```python
from build123d import *

# Parameters (mm, degrees)
EXTRUDE_1_DEPTH          = 1
EXTRUDE_2_DEPTH          = 1
SKETCH_5_W               = 95.882599
SKETCH_5_H               = 27.8428
EXTRUDE_3_DEPTH          = 2
CUT_EXTRUDE_1_DEPTH      = 100.923442209
CUT_EXTRUDE_1_DEPTH_BACK = 100.923442209
SKETCH_6_R               = 5
CUT_EXTRUDE_2_DEPTH      = 100.923442209
CUT_EXTRUDE_2_DEPTH_BACK = 100.923442209
SKETCH_7_R               = 1.35
SKETCH_8_W               = 95.882599
SKETCH_8_H               = 20
EXTRUDE_4_DEPTH          = 2
EXTRUDE_5_DEPTH          = 1
SKETCH_10_W              = 40
SKETCH_10_H              = 120
EXTRUDE_6_DEPTH          = 2
EXTRUDE_START            = -3
EXTRUDE_7_DEPTH          = 3
SKETCH_12_W              = 5
SKETCH_12_H              = 123
EXTRUDE_8_DEPTH          = 1
EXTRUDE_9_OUTLINE_W      = 95.901549254
EXTRUDE_9_OUTLINE_H      = 3
EXTRUDE_9_OUTLINE_W_2    = 95.885
EXTRUDE_9_OUTLINE_H_2    = 2
EXTRUDE_9_DEPTH          = 2
EXTRUDE_START_2          = -1
EXTRUDE_9_2_OUTLINE_W    = 95.885
EXTRUDE_9_2_OUTLINE_H    = 2
EXTRUDE_9_2_DEPTH        = 1
CUT_EXTRUDE_3_DEPTH      = 177.247383378
CUT_EXTRUDE_3_DEPTH_BACK = 177.247383378
SKETCH_16_R              = 1.35
SKETCH_17_W              = 30
SKETCH_17_H              = 70
EXTRUDE_10_DEPTH         = 2
EXTRUDE_11_DEPTH         = 3


# Read off the part's stored shape, not the designer's step: 凸台-拉伸9
with BuildPart() as part:
    # 草图3 → 凸台-拉伸1 (new body)
    with BuildSketch(Plane(origin=(0, 0, 0), x_dir=(1, 0, 0), z_dir=(0, 1, 0))):
        with BuildLine():
            Line((41.882488294, 21.631498957), (31.610829647, 15.243028334))
            ThreePointArc((31.610829647, 15.243028334), (31.350600602, 14.569512784), (31.613242469, 13.896934459))
            Line((31.613242469, 13.896934459), (40.546880152, 8.234769731))
            ThreePointArc((40.546880152, 8.234769731), (44.573930655, 7.017936995), (48.601204689, 8.234029718))
            Line((48.601204689, 8.234029718), (57.364385058, 13.822144736))
            ThreePointArc((57.364385058, 13.822144736), (57.798599734, 14.63340346), (57.366705056, 15.44589967))
            Line((57.366705056, 15.44589967), (47.51874726, 21.632437259))
            ThreePointArc((47.51874726, 21.632437259), (44.700511427, 22.270800367), (41.882488294, 21.631498957))
        make_face()
    extrude(amount=EXTRUDE_1_DEPTH)

    # 草图4 → 凸台-拉伸2 (add)
    with BuildSketch(Plane.XZ):
        with BuildLine():
            Line((49.96883361, -25.998027869), (60.064619869, -19.655803167))
            ThreePointArc((60.064619869, -19.655803167), (62.798594558, -14.643390815), (60.079038247, -9.623140954))
            Line((60.079038247, -9.623140954), (51.324268762, -4.040389399))
            ThreePointArc((51.324268762, -4.040389399), (44.577632655, -2.01793734), (37.829997654, -4.03705422))
            Line((37.829997654, -4.03705422), (28.614522584, -9.877848279))
            ThreePointArc((28.614522584, -9.877848279), (26.350608769, -14.582124379), (28.631489707, -19.27819737))
            Line((28.631489707, -19.27819737), (39.443234024, -26.002574933))
            ThreePointArc((39.443234024, -26.002574933), (44.706582673, -27.270799381), (49.96883361, -25.998027869))
        make_face()
    extrude(amount=EXTRUDE_2_DEPTH)

    # 草图5 → 凸台-拉伸3 (add)
    with BuildSketch(Plane.XZ.offset(1)):
        with Locations((47.9412995, -13.9214)):
            Rectangle(SKETCH_5_W, SKETCH_5_H)
    extrude(amount=EXTRUDE_3_DEPTH)

    # 草图6 → 切除-拉伸1 (cut, two sides: drawn at the far end of the back side and taken through both)
    with BuildSketch(Plane.XZ.offset(3).offset(-CUT_EXTRUDE_1_DEPTH_BACK)):
        with Locations(Location((16.25, -19.8, 0), (0, 0, 270))):
            Circle(SKETCH_6_R)
    extrude(amount=CUT_EXTRUDE_1_DEPTH + CUT_EXTRUDE_1_DEPTH_BACK, mode=Mode.SUBTRACT)

    # 草图7 → 切除-拉伸2 (cut, two sides: drawn at the far end of the back side and taken through both)
    with BuildSketch(Plane(origin=(0, 1, 0), x_dir=(1, 0, 0), z_dir=(0, 1, 0)).offset(-CUT_EXTRUDE_2_DEPTH_BACK)):
        with Locations(Location((37.074600168, 14.583340303, 0), (0, 0, 270))):
            Circle(SKETCH_7_R)
        with Locations(Location((52.074600168, 14.619575942, 0), (0, 0, 270))):
            Circle(SKETCH_7_R)
    extrude(amount=CUT_EXTRUDE_2_DEPTH + CUT_EXTRUDE_2_DEPTH_BACK, mode=Mode.SUBTRACT)

    # 草图8 → 凸台-拉伸4 (add)
    with BuildSketch(Plane(origin=(0, -1, 0), x_dir=(1, 0, 0), z_dir=(0, 1, 0))):
        with Locations((47.9412995, -10)):
            Rectangle(SKETCH_8_W, SKETCH_8_H)
    extrude(amount=-EXTRUDE_4_DEPTH)

    # 草图9 → 凸台-拉伸5 (add)
    with BuildSketch(Plane(origin=(0, -1, 0), x_dir=(1, 0, 0), z_dir=(0, 1, 0))):
        Polygon((0, 0), (0, 4), (95.882599, 4), (95.882599, 0), (95.898271126, -2), (-0.002401, -2), align=None)
    extrude(amount=EXTRUDE_5_DEPTH)

    # 草图10 → 凸台-拉伸6 (add)
    with BuildSketch(Plane(origin=(0, -1, 0), x_dir=(1, 0, 0), z_dir=(0, 1, 0))):
        with Locations((75.882599, 87.8428)):
            Rectangle(SKETCH_10_W, SKETCH_10_H)
    extrude(amount=-EXTRUDE_6_DEPTH)

    # 草图11 → 凸台-拉伸7 (add)
    with BuildSketch(Plane.XZ.offset(3).offset(EXTRUDE_START)):
        Polygon((-0.002401, -27.8428), (-0.002401, -30.8428), (55.882599, -30.8428), (55.882599, -27.8428), (55.882599, -24.8428), (0, -24.8428), align=None)
    extrude(amount=EXTRUDE_7_DEPTH)

    # 草图12 → 凸台-拉伸8 (add)
    with BuildSketch(Plane(origin=(0, -1, 0), x_dir=(1, 0, 0), z_dir=(0, 1, 0))):
        with Locations((58.382599, 86.3428)):
            Rectangle(SKETCH_12_W, SKETCH_12_H)
    extrude(amount=EXTRUDE_8_DEPTH)

    # 凸台-拉伸9 outline → 凸台-拉伸9 (add)
    with BuildSketch(Plane(origin=(0, 0, 0), x_dir=(1, 0, 0), z_dir=(0, 1, 0))):
        with Locations((47.948373627, -2.4702)):
            Rectangle(EXTRUDE_9_OUTLINE_W, EXTRUDE_9_OUTLINE_H)
        with Locations((47.940099, 29.8428)):
            Rectangle(EXTRUDE_9_OUTLINE_W_2, EXTRUDE_9_OUTLINE_H_2)
    extrude(amount=EXTRUDE_9_DEPTH)

    # Extrude 9 2 outline → Extrude 9 2 (add)
    with BuildSketch(Plane(origin=(0, 0, 0), x_dir=(1, 0, 0), z_dir=(0, 1, 0)).offset(EXTRUDE_START_2)):
        with Locations((47.940099, 29.8428)):
            Rectangle(EXTRUDE_9_2_OUTLINE_W, EXTRUDE_9_2_OUTLINE_H)
    extrude(amount=EXTRUDE_9_2_DEPTH)

    # 草图16 → 切除-拉伸3 (cut, two sides: drawn at the far end of the back side and taken through both)
    with BuildSketch(Plane(origin=(0, -1, 0), x_dir=(1, 0, 0), z_dir=(0, 1, 0)).offset(-CUT_EXTRUDE_3_DEPTH_BACK)):
        with Locations(Location((19.997599, -10, 0), (0, 0, 270))):
            Circle(SKETCH_16_R)
        with Locations(Location((26.997599, -10, 0), (0, 0, 270))):
            Circle(SKETCH_16_R)
    extrude(amount=CUT_EXTRUDE_3_DEPTH + CUT_EXTRUDE_3_DEPTH_BACK, mode=Mode.SUBTRACT)

    # 草图17 → 凸台-拉伸10 (add)
    with BuildSketch(Plane(origin=(0, -1, 0), x_dir=(1, 0, 0), z_dir=(0, 1, 0))):
        with Locations((110.882599, 112.8428)):
            Rectangle(SKETCH_17_W, SKETCH_17_H)
    extrude(amount=-EXTRUDE_10_DEPTH)

    # 草图18 → 凸台-拉伸11 (add)
    with BuildSketch(Plane(origin=(0, -1, 0), x_dir=(1, 0, 0), z_dir=(0, 1, 0))):
        Polygon((95.882599, 30.8428), (95.882599, 77.8428), (125.882599, 77.8428), (125.882599, 80.8428), (92.882599, 80.8428), (92.882599, 31.8428), (60.882599, 31.8428), (60.882599, 144.8428), (125.882599, 144.8428), (125.882599, 147.8428), (55.882599, 147.8428), (55.882599, 30.8428), (60.882599, 30.8428), align=None)
    extrude(amount=EXTRUDE_11_DEPTH)


solid = part.part
```
Check sheet for the modelled part. Datum: model origin and axes. Units: mm. A direction names the side the tool comes from. Give positions to 0.01 mm unless a question says otherwise; leave off trailing zeros. Loops run counter-clockwise (first coordinate to the right, second up) from the corner with the lowest first, then second, coordinate; pieces in that order, holes last. Notation, with made-up numbers: (-6, -28.5) - (28, -28.5) arc R16 cw to (28, -5.5) - close; hole circle Ø9 at (3.25, 49). An arc over 180 degrees is marked (long way). One line per question, with ' | ' between items. Start each with the question number.
1. Gauge pin test, flat ends, axial feed: pin 1 Ø6 at (x, z) = (16.25, -19.8) entering from +Y; pin 2 Ø2.5 at (x, y) = (37.5, -1) entering from -Z; pin 3 Ø20 at (x, z) = (83.5, -18.5) entering from +Y; pin 4 Ø1.5 at (y, z) = (-1.5, -87) entering from -X. Record the tip position at first contact, or that the pin passes through.
2. Draft check along Z on faces 1 (the flat face through (52.92, 0.49, -10.99)), 2 (the flat face through (91, -1, -147.843)), 3 (the flat face through (76, -3, -65)). Enter one of: released by +Z, released by -Z, zero draft, split by the parting line, or undercut.
3. Cross-section at C-C, the plane x = 108.5. Enter the section's corners in (y, z).
4. Cross-section at A-A, the plane x = 16.25. Enter the section's corners in (y, z).
5. Cross-section at B-B, the plane z = -72. Enter the section's corners in (x, y).
6. Set-up check for faces 4 (the flat face through (52.512, 0.493, -18.496)), 5 (the flat face through (111, -1, -77.843)), 6 (the flat face through (44, 1, -15)), 7 (the flat face through (36.819, 0.493, -18.482)), 8 (the flat face through (55.883, -1, -90)): record each of +Z, -Z, +X, -X, +Y, -Y from which the full face is reachable in a straight line by a thin tool's end or side.
7. Material ranges on line 1 along Z through (x, y) = (56.5, 0.7); line 2 along Z through (x, y) = (71.5, 1.5); line 3 along Z through (x, y) = (52, -1.05), recorded low to high. Write a range as [from, to].
Check result:
1) pin 1: passes through | pin 2: stops at z = -30.84 | pin 3: stops at y = -1 | pin 4: stops at x = 55.88
2) face 1: undercut | face 2: released by -Z | face 3: zero draft
3) outline: (-3, -147.84) - (2, -147.84) - (2, -144.84) - (-1, -144.84) - (-1, -80.84) - (2, -80.84) - (2, -77.84) - (-3, -77.84) - close
4) outline: (-3, -30.84) - (2, -30.84) - (2, -28.84) - (0, -28.84) - (0, -24.84) - (-1, -24.84) - (-1, -24.8) - (-3, -24.8) - close; (-3, -14.8) - (-1, -14.8) - (-1, -4) - (0, -4) - (0, 0.97) - (2, 0.97) - (2, 3.97) - (0, 3.97) - (0, 2) - (-1, 2) - (-1, 20) - (-3, 20) - close
5) outline: (55.88, -3) - (95.88, -3) - (95.88, 2) - (92.88, 2) - (92.88, -1) - (60.88, -1) - (60.88, 2) - (55.88, 2) - close
6) face 4: +X, +Y | face 5: +Z, +X, +Y, -Y | face 6: +X, -X, +Y | face 7: -X, +Y | face 8: -Z, -X, +Y, -Y
7) line 1: z = [-147.84, -28.84], [-15.99, -13.27], [0.97, 3.97] | line 2: z = [-147.84, -144.84], [-31.84, -28.84], [0.97, 3.97] | line 3: z = [-30.84, -15.97], [-13.27, 20]
